```python
from build123d import *

# Parameters (mm, degrees)
FRONT_COVER_REFERENCE_START = 58.5
SKETCH_1_R                  = 78.5
SKETCH_1_R_2                = 17.5
FRONT_COVER_REFERENCE_DEPTH = 2.5
SKETCH_2_R                  = 2.25
THROUGH_HOLES_DEPTH         = 100


with BuildPart() as part:
    # Эскиз1 → Front_cover_reference (new body)
    with BuildSketch(Plane.XY.offset(FRONT_COVER_REFERENCE_START)):
        Circle(SKETCH_1_R)
        Circle(SKETCH_1_R_2, mode=Mode.SUBTRACT)
    extrude(amount=FRONT_COVER_REFERENCE_DEPTH)

    # Эскиз2 → Through_holes (cut, symmetric)
    with BuildSketch(Plane.XY):
        with Locations((38.154070138, 10.223352282)):
            Circle(SKETCH_2_R)
        with Locations((10.223352282, 38.154070138)):
            Circle(SKETCH_2_R)
        with Locations((-27.930717857, 27.930717857)):
            Circle(SKETCH_2_R)
        with Locations((-38.154070138, -10.223352282)):
            Circle(SKETCH_2_R)
        with Locations((-10.223352282, -38.154070138)):
            Circle(SKETCH_2_R)
        with Locations((27.930717857, -27.930717857)):
            Circle(SKETCH_2_R)
    extrude(amount=THROUGH_HOLES_DEPTH, both=True, mode=Mode.SUBTRACT)


solid = part.part
```
Check sheet for the modelled part. Datum: model origin and axes. Units: mm. Coordinates: 2 decimals unless noted, no trailing zeros. Write each loop counter-clockwise with the first axis right and the second up, starting at its lowest first coordinate (ties: lowest second). Pieces come first, ordered by that corner, then holes. Notation, with made-up numbers: M 47.5,-8 L 55.5,-8 A33 cw 55.5,27 Z; hole C 87,49 d1. An arc over 180 degrees is marked long. Write item = value, one per line. Start each with the question number.
1. Sectioned sample at A-A (x = 0). Record the cut outline in (y, z), then the cut area to 3 significant figures.
2. Sectioned sample at D-D (x = -66.5). Record the cut outline in (y, z), then the cut area to 3 significant figures.
3. Thickness scan on probe 1 along Y at (x, z) = (10.5, 60.45); probe 2 along Y at (x, z) = (-8.5, 60.5). Record the ranges inside material, lowest first.
4. Sectioned sample at C-C (z = 59.3). Record the cut outline in (x, y).
5. Mould release check, pull along Y, two halves, no side actions. Record for faces 1 (the cylindrical face through (-78.424, 3.451, 59.732)), 2 (the cylindrical face through (-36.076, -11.085, 59.732)), 3 (the flat face through (-1, 19, 61)): pulls with the +Y half, pulls with the -Y half, needs draft (parallel to the pull), parting line crosses it, or undercut.
The answers:
q1.outline = M -78.5,58.5 L -17.5,58.5 L -17.5,61 L -78.5,61 Z; M 17.5,58.5 L 78.5,58.5 L 78.5,61 L 17.5,61 Z
q1.area = 305 mm²
q2.outline = M -41.71,58.5 L 41.71,58.5 L 41.71,61 L -41.71,61 Z
q2.area = 209 mm²
q3.probe_1 = -77.79 to -14, 14 to 35.92, 40.39 to 77.79
q3.probe_2 = -78.04 to -39.6, -36.71 to -15.3, 15.3 to 78.04
q4.outline = C 0,0 d157; hole C -38.15,-10.22 d4.5; hole C -27.93,27.93 d4.5; hole C 0,0 d35; hole C -10.22,-38.15 d4.5; hole C 10.22,38.15 d4.5; hole C 27.93,-27.93 d4.5; hole C 38.15,10.22 d4.5
q5.face_1 = parting line crosses it
q5.face_2 = undercut
q5.face_3 = needs draft
